Autodesk Inventor part; units mm, degrees
ref_plane "YZ Plane" through (0, 0, 0) normal (1, 0, 0) x (0, 1, 0)
ref_plane "XZ Plane" through (0, 0, 0) normal (0, 1, 0) x (-1, 0, 0)
ref_plane "XY Plane" through (0, 0, 0) normal (0, 0, 1) x (1, 0, 0)
ref_plane "РабПлоскость1" through (0, 0, 0) normal (0, 0, 1) x (1, 0, 0)
sketch "Эскиз1" plane through (0, 0, 0) normal (0, 0, 1) x (1, 0, 0)
  line L0 (-54.6061, 570.3445) -> (-45.6061, 570.3445)
  line L1 (-45.6061, 570.3445) -> (-45.6061, 587.3445)
  line L2 (-45.6061, 587.3445) -> (-54.6061, 587.3445)
  line L3 (-54.6061, 587.3445) -> (-54.6061, 627.3645)
  line L4 (-54.6061, 627.3645) -> (-114.6061, 627.3645)
  line L5 (-114.6061, 627.3645) -> (-114.6061, 587.3445)
  line L6 (-114.6061, 587.3445) -> (-123.6061, 587.3445)
  line L7 (-123.6061, 587.3445) -> (-123.6061, 570.3445)
  line L8 (-123.6061, 570.3445) -> (-114.6061, 570.3445)
  line L9 (-114.6061, 570.3445) -> (-114.6061, 557.3645)
  line L10 (-114.6061, 557.3645) -> (-54.6061, 557.3645)
  line L11 (-54.6061, 557.3645) -> (-54.6061, 570.3445)
  line L12 (-48.6061, 575.3445) -> (-51.6061, 575.3445)
  line L13 (-51.6061, 575.3445) -> (-51.6061, 582.3445)
  line L14 (-51.6061, 582.3445) -> (-48.6061, 582.3445)
  line L15 (-48.6061, 582.3445) -> (-48.6061, 575.3445)
  line L16 (-117.6061, 582.3445) -> (-117.6061, 575.3445)
  line L17 (-117.6061, 575.3445) -> (-120.6061, 575.3445)
  line L18 (-120.6061, 575.3445) -> (-120.6061, 582.3445)
  line L19 (-120.6061, 582.3445) -> (-117.6061, 582.3445)
  circle A0 centre (-97.1061, 577.3245) radius 2.575
  circle A1 centre (-72.1061, 577.3245) radius 2.575
  circle A2 centre (-72.1061, 617.3645) radius 2.575
  circle A3 centre (-97.1061, 617.3645) radius 2.575
  circle A4 centre (-109.6061, 560.8645) radius 1.5
  circle A5 centre (-59.6061, 560.8645) radius 1.5
  circle A6 centre (-106.1061, 572.3645) radius 1
  circle A7 centre (-63.1061, 572.3645) radius 1
  circle A8 centre (-106.1061, 587.3645) radius 1
  circle A9 centre (-63.1061, 587.3645) radius 1
  circle A10 centre (-106.1061, 602.3645) radius 1
  circle A11 centre (-63.1061, 602.3645) radius 1
  circle A12 centre (-106.1061, 617.3645) radius 1
  circle A13 centre (-63.1061, 617.3645) radius 1
  line L20 (-59.6061, 627.3645) -> (-54.6061, 627.3645)
  line L21 (-54.6061, 627.3645) -> (-54.6061, 557.3645)
  line L22 (-54.6061, 557.3645) -> (-59.6061, 557.3645)
  line L23 (-59.6061, 557.3645) -> (-59.6061, 627.3645)
  line L24 (-54.6061, 557.3645) -> (-114.6061, 557.3645)
  line L25 (-114.6061, 557.3645) -> (-114.6061, 565.3645)
  line L26 (-114.6061, 565.3645) -> (-54.6061, 565.3645)
  line L27 (-54.6061, 565.3645) -> (-54.6061, 557.3645)
  line L28 (-114.6061, 557.3645) -> (-109.6061, 557.3645)
  line L29 (-109.6061, 557.3645) -> (-109.6061, 627.3645)
  line L30 (-109.6061, 627.3645) -> (-114.6061, 627.3645)
  line L31 (-114.6061, 627.3645) -> (-114.6061, 557.3645)
  circle A14 centre (-59.6061, 560.8645) radius 1.5
  circle A15 centre (-109.6061, 560.8645) radius 1.5
  point P0 (0, 0)
  point P1 (-59.6061, 565.3645)
  point P2 (-109.6061, 565.3645)
  dimension "d0" = 5
  dimension "d1" = 5
  dimension "d2" = 8
extrude "Выдавливание1" add sketch "Эскиз1" along normal blind 3.65 contours L11 L26 L23 L4 L3 L21 | L11 L10 L23 A5 L26 | L23 A5 L10 L29 A4 L26 | L29 A4 L10 L9 L26 | L26 L9 L31 L5 L4 L29
fillet "Сопряжение грани1" radius 5 1 edges at (-109.6061, 565.3645, 1.825)
fillet "Сопряжение грани2" radius 5 1 edges at (-59.6061, 565.3645, 1.825)
fillet "Сопряжение грани3" radius 5 1 edges at (-59.6061, 627.3645, 1.825)
fillet "Сопряжение грани4" radius 5 1 edges at (-114.6061, 627.3645, 1.825)
feature "Сопряжение грани5" [suppressed]
feature "Сопряжение грани6" [suppressed]
fillet "Сопряжение грани7" radius 5 1 edges at (-54.6061, 557.3645, 1.825)
fillet "Сопряжение грани8" radius 5 1 edges at (-114.6061, 557.3645, 1.825)
properties part number "соединялка"
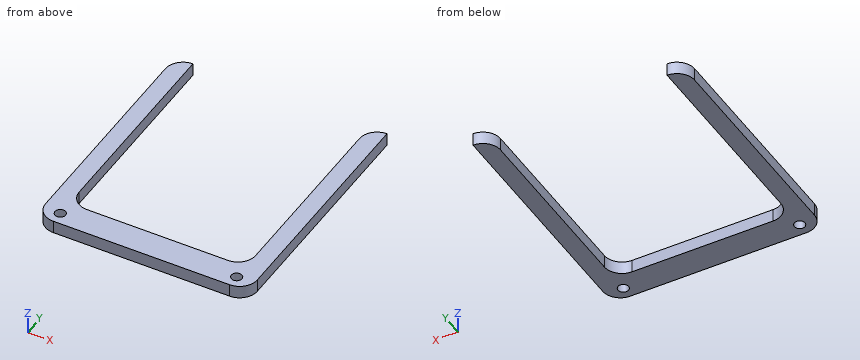
The model under review builds one solid part; all positions refer to its coordinate system, in mm. Round coordinates to 2 decimals unless told otherwise and drop trailing zeros. Loops run counter-clockwise (first coordinate to the right, second up) from the corner with the lowest first, then second, coordinate; pieces in that order, holes last.
Item 1: Take a section at B-B (z = 1.15). Give the number of separate pieces and of enclosed holes in the cut face, then the cut area to 3 significant figures.
Determined:
separate pieces: 1
enclosed holes: 2
area: 1,080 mm2
Item 2: Take a section at C-C (x = -81). Write out the cut boundary in (y, z).
Determined:
outline: (557.36, 0) - (565.36, 0) - (565.36, 3.65) - (557.36, 3.65) - close
Item 3: Take a section at A-A (y = 577). Write out the cut boundary in (x, z).
Determined:
outline: (-114.61, 0) - (-109.61, 0) - (-109.61, 3.65) - (-114.61, 3.65) - close; (-59.61, 0) - (-54.61, 0) - (-54.61, 3.65) - (-59.61, 3.65) - close
Item 4: Clearance check with a flat-ended pin moving along its axis: pin 1 Ø1.8 at (x, z) = (-91, 2) entering from +Y. State where the tip first meets the part, or that it passes through.
Determined:
pin 1: stops at y = 565.36
Item 5: For line 1 (X direction, y = 600, z = 3.2); line 2 (Y direction, x = -74, z = 1.4); line 3 (Y direction, x = -62, z = 3), list the stretches that pass through material, from the lowest coordinate up.
Determined:
line 1: x = -114.61 to -109.61, -59.61 to -54.61
line 2: y = 557.36 to 565.36
line 3: y = 557.36 to 566.1
